from build123d import *

# Parameters (mm, degrees)
CHAMFER1_SIZE      = 0.4
CUT_EXTRUDE1_START = -2.4000001
CUT_EXTRUDE1_DEPTH = 3.4000001
FILLET1_R          = 0.2


with BuildPart() as part:
    # Sketch1 → Revolve1 (revolve)
    with BuildSketch(Plane(origin=(0, 0, 0), x_dir=(0, 0, -1), z_dir=(1, 0, 0)), mode=Mode.PRIVATE) as revolve1_sk:
        with BuildLine():
            Line((25, 0), (25, 2.5))
            Line((25, 2.5), (0, 2.5))
            Line((0, 2.5), (0, 4.75))
            Line((0, 4.75), (-0.5, 4.75))
            ThreePointArc((-0.5, 4.75), (-2.374208166, 4.080480498), (-3.4, 2.375))
            Line((-3.4, 2.375), (-3.4, 0))
            Line((-3.4, 0), (25, 0))
        make_face()
    revolve(revolve1_sk.sketch.rotate(Axis((0, 0, 30.809969789), (0, 0, -1)), 90), axis=Axis((0, 0, 30.809969789), (0, 0, -1)))

    # Chamfer1
    chamfer1_edges = [part.edges().sort_by_distance(p)[0] for p in [
        (-2.5, 0, -25),
    ]]
    chamfer(chamfer1_edges, length=CHAMFER1_SIZE)

    # Sketch2 → Cut-Revolve1 (revolve, cut)
    with BuildSketch(Plane(origin=(0, 0, 0), x_dir=(0, 0, -1), z_dir=(1, 0, 0)), mode=Mode.PRIVATE) as cut_revolve1_sk:
        Polygon((-3.4, 0), (-3.4, 1.5), (-1, 1.5), (-0.133974596, 0), align=None)
    revolve(cut_revolve1_sk.sketch.rotate(Axis((0, 0, 2.452500839), (0, 0, -1)), 90), axis=Axis((0, 0, 2.452500839), (0, 0, -1)), mode=Mode.SUBTRACT)

    # Cut-Extrude1: read off the stored shape, not the designer's step
    # Cut-Extrude1 outline → Cut-Extrude1 (cut)
    with BuildSketch(Plane.XY.offset(3.4).offset(CUT_EXTRUDE1_START)):
        with BuildLine():
            Line((1.5, 0), (1.5, 0.866025404))
            Line((1.5, 0.866025404), (0.750000011, 1.299038099))
            ThreePointArc((0.750000011, 1.299038099), (1.299038109, 0.749999994), (1.5, 0))
        make_face()
        with BuildLine():
            ThreePointArc((-0.749999993, 1.29903811), (1e-08, 1.5), (0.750000011, 1.299038099))
            Line((0.750000011, 1.299038099), (0, 1.732050808))
            Line((0, 1.732050808), (-0.749999993, 1.29903811))
        make_face()
        with BuildLine():
            Line((1.5, -0.866025404), (1.5, 0))
            ThreePointArc((1.5, 0), (1.299038107, -0.749999997), (0.750000005, -1.299038103))
            Line((0.750000005, -1.299038103), (1.5, -0.866025404))
        make_face()
        with BuildLine():
            ThreePointArc((-1.5, 0), (-1.299038104, 0.750000003), (-0.749999993, 1.29903811))
            Line((-0.749999993, 1.29903811), (-1.5, 0.866025404))
            Line((-1.5, 0.866025404), (-1.5, 0))
        make_face()
        with BuildLine():
            Line((0, -1.732050808), (0.750000005, -1.299038103))
            ThreePointArc((0.750000005, -1.299038103), (3e-09, -1.5), (-0.75, -1.299038106))
            Line((-0.75, -1.299038106), (0, -1.732050808))
        make_face()
        with BuildLine():
            ThreePointArc((-0.75, -1.299038106), (-1.299038106, -0.75), (-1.5, 0))
            Line((-1.5, 0), (-1.5, -0.866025404))
            Line((-1.5, -0.866025404), (-0.75, -1.299038106))
        make_face()
    extrude(amount=CUT_EXTRUDE1_DEPTH, mode=Mode.SUBTRACT)

    # Cut-Extrude1 2 outline → Cut-Extrude1 2 (revolve)
    with BuildSketch(Plane.XZ):
        Polygon((1.732050837, 1.133974613), (1.499999957, 0.999999975), (1.732050808, 0.9999999), align=None)
    revolve(axis=Axis((0, 0, 0), (0, 0, 1)))

    # Fillet1
    fillet1_edges = [part.edges().sort_by_distance(p)[0] for p in [
        (-2.5, 0, 0),
    ]]
    fillet(fillet1_edges, radius=FILLET1_R)


solid = part.part
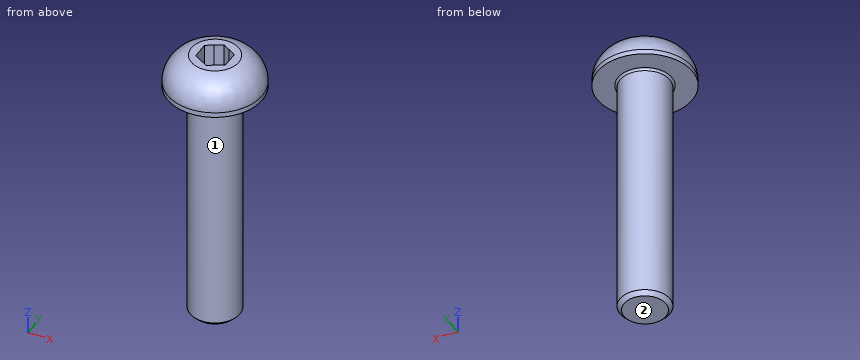
CAD build for the part. Positions are in the model's coordinates, mm. Face numbers are marked on the shaded views. A direction names the side the tool comes from. Coordinates: 2 decimals unless noted, no trailing zeros. Write each loop counter-clockwise with the first axis right and the second up, starting at its lowest first coordinate (ties: lowest second). Pieces come first, ordered by that corner, then holes. Notation, with made-up numbers: (-39, 60) - (-35, 60) arc R20 ccw to (-35, 68) - close; hole circle Ø3 at (52, 88). An arc over 180 degrees is marked (long way). Use a Markdown table: item, result. Add a question column.
Item 1: 3-axis set-ups, long thin cutter, end or side, ignore diameter. For the marked faces 1 and 2: which of +Z, -Z, +X, -X, +Y, -Y reach the whole face in a straight line?
Item 2: Band-saw the part on A-A, the plane z = -0.5. Give the cut face in (x, y), and give its area (3 significant figures).
Item 3: Drill centre lines: L1, parallel to Y at x = 0, z = -19.75; L2, parallel to X at y = 1.5, z = -18.5; L3, parallel to X at y = 0.25, z = -3.25. Where is each one in solid material? Low to high. Write a range as from..to.
Item 4: Flat gauge pins, fed straight in: pin 1 (1.9 mm diameter, centred on y = -0.5, z = 2.5, fed in from +X); pin 2 (3 mm diameter, centred on x = -1, z = -15, fed in from +Y); pin 3 (1 mm diameter, centred on x = 1, z = -7.5, fed in from -Y). Where does each tip first touch, or does it go through?
Numbers:
| question | item | result |
|---|---|---|
| 1 | face 1 | -Z |
| 1 | face 2 | -Z, +X, -X, +Y, -Y |
| 2 | outline | circle Ø5 at (0, 0) |
| 2 | area | 19.6 mm2 |
| 3 | L1 | -2.5..2.5 |
| 3 | L2 | -2..2 |
| 3 | L3 | -2.49..2.49 |
| 4 | pin 1 | x = 4.54 |
| 4 | pin 2 | y = 2.5 |
| 4 | pin 3 | y = -2.45 |
